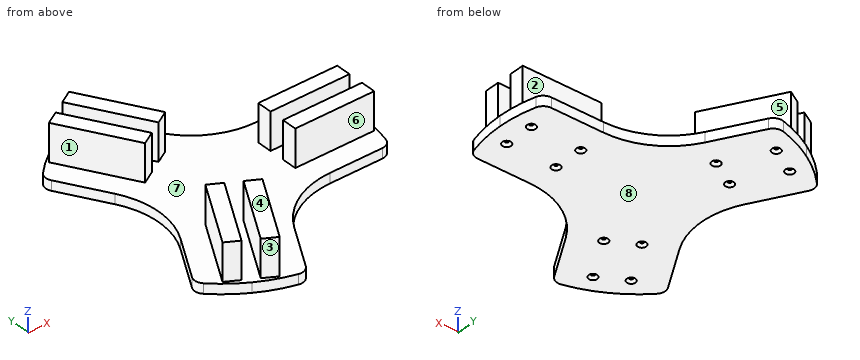
```python
from build123d import *

# Parameters (mm, degrees)
F0_W           = 101.6
F0_H           = 19.05
F1_DEPTH       = 12.7
F2_DEPTH       = 9.525
F3_DEPTH       = 50.8
F4_D           = 4.7625
F4_DEPTH       = 12.7
F4_CSINK_D     = 11.0998
F4_CSINK_ANGLE = 90
F4_TIP         = 1.4307993491


with BuildPart() as f1:
    # F0 (on Top) → F1 (new body)
    with BuildSketch(Plane.XY):
        with BuildLine():
            Line((-88.9, -153.9793167929), (0, 0))
            Line((0, 0), (-88.9, 153.9793167929))
            ThreePointArc((-88.9, 153.9793167929), (-108.9975516555, 140.471967784), (-127.0733991266, 124.3591220394))
            ThreePointArc((-127.0733991266, 124.3591220394), (-130.596841253, 117.066025685), (-128.9952503885, 109.126327608))
            Line((-128.9952503885, 109.126327608), (-95.3205294432, 50.8))
            ThreePointArc((-95.3205294432, 50.8), (-81.7087104677, 0), (-95.3205294432, -50.8))
            Line((-95.3205294432, -50.8), (-128.9952503885, -109.126327608))
            ThreePointArc((-128.9952503885, -109.126327608), (-130.596841253, -117.066025685), (-127.0733991266, -124.3591220394))
            ThreePointArc((-127.0733991266, -124.3591220394), (-108.9975516555, -140.471967784), (-88.9, -153.9793167929))
        make_face()
        Polygon((-60.1282869611, -46.7410218803), (-43.630503019, -56.2660218803), (-94.430503019, -144.2542029048), (-110.9282869611, -134.7292029048), align=None, mode=Mode.SUBTRACT)
        Polygon((-43.630503019, 56.2660218803), (-60.1282869611, 46.7410218803), (-110.9282869611, 134.7292029048), (-94.430503019, 144.2542029048), align=None, mode=Mode.SUBTRACT)
        with BuildLine():
            Line((0, 0), (177.8, 0))
            ThreePointArc((177.8, 0), (176.1510684483, 24.1586647919), (171.2348584417, 47.8692307692))
            ThreePointArc((171.2348584417, 47.8692307692), (166.6805727898, 54.5671693366), (159.0037971245, 57.15))
            Line((159.0037971245, 57.15), (91.6543552339, 57.15))
            ThreePointArc((91.6543552339, 57.15), (40.8543552339, 70.7618189755), (3.6661742094, 107.95))
            Line((3.6661742094, 107.95), (-30.008546736, 166.276327608))
            ThreePointArc((-30.008546736, 166.276327608), (-36.0837315368, 171.6331950216), (-44.1614593151, 172.2283528086))
            ThreePointArc((-44.1614593151, 172.2283528086), (-67.1535167928, 164.630632576), (-88.9, 153.9793167929))
            Line((-88.9, 153.9793167929), (0, 0))
        make_face()
        Polygon((-10.4147688666, 75.4431349345), (-26.9125528087, 65.9181349345), (-77.7125528087, 153.906315959), (-61.2147688666, 163.431315959), align=None, mode=Mode.SUBTRACT)
        with Locations((121.3430558277, 19.1771130542)):
            Rectangle(F0_W, F0_H, mode=Mode.SUBTRACT)
        with BuildLine():
            ThreePointArc((159.0037971245, -57.15), (166.6805727898, -54.5671693366), (171.2348584417, -47.8692307692))
            ThreePointArc((171.2348584417, -47.8692307692), (176.1510684483, -24.1586647919), (177.8, 0))
            Line((177.8, 0), (0, 0))
            Line((0, 0), (-88.9, -153.9793167929))
            ThreePointArc((-88.9, -153.9793167929), (-67.1535167928, -164.630632576), (-44.1614593151, -172.2283528086))
            ThreePointArc((-44.1614593151, -172.2283528086), (-36.0837315368, -171.6331950216), (-30.008546736, -166.276327608))
            Line((-30.008546736, -166.276327608), (3.6661742094, -107.95))
            ThreePointArc((3.6661742094, -107.95), (40.8543552339, -70.7618189755), (91.6543552339, -57.15))
            Line((91.6543552339, -57.15), (159.0037971245, -57.15))
        make_face()
        Polygon((-26.9125528087, -65.9181349345), (-10.4147688666, -75.4431349345), (-61.2147688666, -163.431315959), (-77.7125528087, -153.906315959), align=None, mode=Mode.SUBTRACT)
        with Locations((121.3430558277, -19.1771130542)):
            Rectangle(F0_W, F0_H, mode=Mode.SUBTRACT)
    extrude(amount=F1_DEPTH)

    # F0 (on Top) → F2 (join)
    with BuildSketch(Plane.XY):
        Polygon((-94.430503019, -144.2542029048), (-43.630503019, -56.2660218803), (-60.1282869611, -46.7410218803), (-110.9282869611, -134.7292029048), align=None)
        Polygon((-61.2147688666, -163.431315959), (-10.4147688666, -75.4431349345), (-26.9125528087, -65.9181349345), (-77.7125528087, -153.906315959), align=None)
        with Locations((121.3430558277, -19.1771130542)):
            Rectangle(F0_W, F0_H)
        with Locations((121.3430558277, 19.1771130542)):
            Rectangle(F0_W, F0_H)
        Polygon((-77.7125528087, 153.906315959), (-26.9125528087, 65.9181349345), (-10.4147688666, 75.4431349345), (-61.2147688666, 163.431315959), align=None)
        Polygon((-110.9282869611, 134.7292029048), (-60.1282869611, 46.7410218803), (-43.630503019, 56.2660218803), (-94.430503019, 144.2542029048), align=None)
    extrude(amount=F2_DEPTH)

    # F3 (add): faces of the model
    f3_faces = [f1.faces().sort_by_distance(p)[0] for p in [
        (-77.2793949901, -95.4976123925, 9.525),
        (-44.0636608377, -114.6747254468, 9.525),
        (121.3430558277, -19.1771130542, 9.525),
        (121.3430558277, 19.1771130542, 9.525),
        (-44.0636608377, 114.6747254468, 9.525),
        (-77.2793949901, 95.4976123925, 9.525),
    ]]
    extrude(f3_faces, amount=F3_DEPTH)

    # F4
    with Locations(Plane(origin=(0, 0, 0), x_dir=(1, 0, 0), z_dir=(0, 0, -1))):
        with Locations((-93.1543949901, 122.9939189627), (-59.9386608377, 142.1710320169), (-28.1886608377, 87.1784188766), (-61.4043949901, 68.0013058224), (89.5930558277, 19.1771130542), (153.0930558277, 19.1771130542), (153.0930558277, -19.1771130542), (89.5930558277, -19.1771130542), (-61.4043949901, -68.0013058224), (-28.1886608377, -87.1784188766), (-59.9386608377, -142.1710320169), (-93.1543949901, -122.9939189627)):
            CounterSinkHole(F4_D / 2, F4_CSINK_D / 2, depth=F4_DEPTH, counter_sink_angle=F4_CSINK_ANGLE)
            with Locations((0, 0, -(F4_DEPTH + F4_TIP / 2))):  # 118° drill point
                Cone(0, F4_D / 2, F4_TIP, mode=Mode.SUBTRACT)


solid = f1.part
```
Geometry: final body of the model. Coordinates: model frame, mm. Face numbers are marked on the shaded views. A direction names the side the tool comes from. Round coordinates to 2 decimals unless told otherwise and drop trailing zeros. Order: outer loops, then holes, each group sorted by start corner. A loop starts at its lowest first (then second) coordinate and runs counter-clockwise, first axis right, second up. Notation, with made-up numbers: M -34.75,32 L -0.75,32 A16 cw -0.75,47 Z; hole C 37.25,-7 d7. An arc over 180 degrees is marked long. Use one line per item in the form item = value. Start each with the question number.
Q1. Pin query (flat end, axial travel): pin 1 Ø5.5 at (x, y) = (89.59, 19.18) entering from -Z; pin 2 Ø4 at (y, z) = (6.5, 36) entering from -X; pin 3 Ø15 at (y, z) = (-23.5, 26.5) entering from +X; pin 4 Ø5.5 at (y, z) = (17, 34) entering from -X. Return the tip coordinate at first contact, or that it passes through.
Q2. Cut plane C-C (x = 77). Return loops of the section in (y, z) (3 decimals), and give its area (3 significant figures).
Q3. Cut plane D-D (x = 21). Return loops of the section in (y, z), and give its area (3 significant figures).
Q4. Cut plane A-A (z = 20). Return loops of the section in (x, y), and give its area (3 significant figures).
Q5. Mould query, pull axis Y, two halves, no side actions, for the marked faces 5, 6, 7 and 8. Classes: +Y half, -Y half, draft (parallel to the pull), parting line (faces both ways), or undercut.
Q6. Cut plane B-B (x = 114). Return loops of the section in (y, z) (3 decimals).
Q7. Material intervals for line 1 (Y direction, x = -52, z = 33.5); line 2 (Y direction, x = -44, z = 51); line 3 (Y direction, x = 106, z = 50.5), sorted ascending. Write a range as [from, to].
Q8. Access query for the marked faces 1, 2, 3 and 4. Directions: +Z, -Z, +X, -X, +Y, -Y. A direction counts if a zero-diameter tool reaches every point of the face in a straight line with its end or side. Return the directions, or none.
Geometry results:
q1.pin_1 = 2.8
q1.pin_2 = through
q1.pin_3 = 172.14
q1.pin_4 = 70.54
q2.outline = M -58.212,0 L 58.212,0 L 58.212,12.7 L 28.702,12.7 L 28.702,60.325 L 9.652,60.325 L 9.652,12.7 L -9.652,12.7 L -9.652,60.325 L -28.702,60.325 L -28.702,12.7 L -58.212,12.7 Z
q2.area = 3,290 mm^2
q3.outline = M -85.74,0 L 85.74,0 L 85.74,12.7 L -85.74,12.7 Z
q3.area = 2,180 mm^2
q4.outline = M -110.93,-134.73 L -94.43,-144.25 L -43.63,-56.27 L -60.13,-46.74 Z; M -110.93,134.73 L -60.13,46.74 L -43.63,56.27 L -94.43,144.25 Z; M -77.71,-153.91 L -61.21,-163.43 L -10.41,-75.44 L -26.91,-65.92 Z; M -77.71,153.91 L -26.91,65.92 L -10.41,75.44 L -61.21,163.43 Z; M 70.54,-28.7 L 172.14,-28.7 L 172.14,-9.65 L 70.54,-9.65 Z; M 70.54,9.65 L 172.14,9.65 L 172.14,28.7 L 70.54,28.7 Z
q4.area = 11,600 mm^2
q5.face_5 = +Y half
q5.face_6 = -Y half
q5.face_7 = undercut
q5.face_8 = draft
q6.outline = M -57.15,0 L 57.15,0 L 57.15,12.7 L 28.702,12.7 L 28.702,60.325 L 9.652,60.325 L 9.652,12.7 L -9.652,12.7 L -9.652,60.325 L -28.702,60.325 L -28.702,12.7 L -57.15,12.7 Z
q7.line_1 = [-147.47, -109.37], [-70.76, -51.43], [51.43, 70.76], [109.37, 147.47]
q7.line_2 = [-133.61, -95.51], [-56.91, -56.05], [56.05, 56.91], [95.51, 133.61]
q7.line_3 = [-28.7, -9.65], [9.65, 28.7]
q8.face_1 = +Z, -X
q8.face_2 = +Z, +X, -X, +Y
q8.face_3 = +Z, -X, -Y
q8.face_4 = +Z, +X, -X, +Y, -Y
